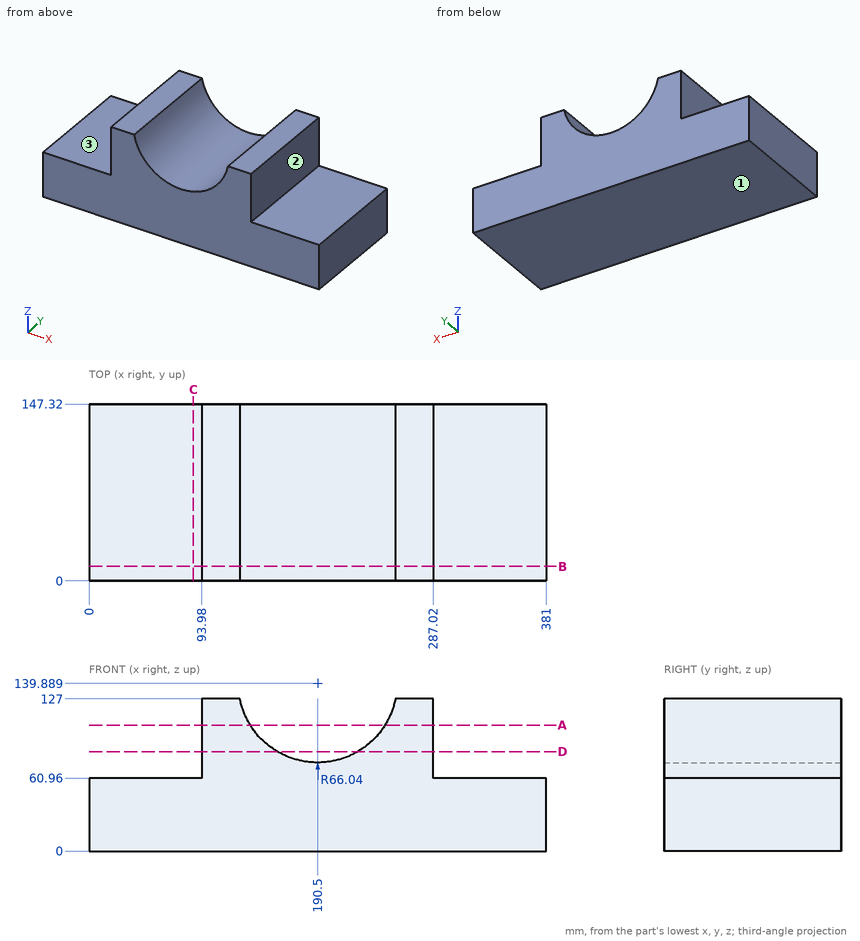
Verification items for this drawing (mm, ordinates from the low corner). A direction names the side the tool comes from. Coordinates: 2 decimals unless noted, no trailing zeros. Order: outer loops, then holes, each group sorted by start corner. A loop starts at its lowest first (then second) coordinate and runs counter-clockwise, first axis right, second up. Notation, with made-up numbers: (65.25, 25.25) - (76.25, 25.25) arc R23 ccw to (76.25, 57.25) - close; hole circle Ø8 at (74.5, 50.25). An arc over 180 degrees is marked (long way). Answer as a JSON object with one key per item and string values. Group by question number.
Item 1: Sectioned sample at C-C, the plane x = 87. Record the cut outline in (y, z).
Item 2: Sectioned sample at D-D, the plane z = 83. Record the cut outline in (x, y), and give its area (3 significant figures).
Item 3: Sectioned sample at B-B, the plane y = 12. Record the cut outline in (x, z).
Item 4: Sectioned sample at A-A, the plane z = 105. Record the cut outline in (x, y).
Item 5: Tool access check on the marked faces 1, 2 and 3. Record the directions out of +Z, -Z, +X, -X, +Y, -Y that give a thin tool (end or side, any length) a straight path to the whole face; none if there is none.
Item 6: Depth check by flat-ended pin: pin 1 Ø4 at (x, y) = (59, 21.5) entering from +Z; pin 2 Ø6 at (y, z) = (18, 68.5) entering from +X; pin 3 Ø20 at (y, z) = (45.5, 95.5) entering from -X. Enter the tip coordinate at first touch or a pass-through.
Item 7: Scan lines: probe 1 along Z at (x, y) = (291, 45); probe 2 along X at (y, z) = (121.5, 108.5); probe 3 along X at (y, z) = (67, 99). Record each from-to range of solid material in increasing order.
Resolved:
{
 "1": {"outline": "(0, 0) - (147.32, 0) - (147.32, 60.96) - (0, 60.96) - close"},
 "2": {"outline": "(93.98, 0) - (156.96, 0) - (156.96, 147.32) - (93.98, 147.32) - close; (224.04, 0) - (287.02, 0) - (287.02, 147.32) - (224.04, 147.32) - close", "area": "18,600 mm^2"},
 "3": {"outline": "(0, 0) - (381, 0) - (381, 60.96) - (287.02, 60.96) - (287.02, 127) - (255.27, 127) arc R66.04 cw to (125.73, 127) - (93.98, 127) - (93.98, 60.96) - (0, 60.96) - close"},
 "4": {"outline": "(93.98, 0) - (134.43, 0) - (134.43, 147.32) - (93.98, 147.32) - close; (246.57, 0) - (287.02, 0) - (287.02, 147.32) - (246.57, 147.32) - close"},
 "5": {"face 1": "-Z, +X, -X, +Y, -Y", "face 2": "+Z, +X, +Y, -Y", "face 3": "+Z, -X, +Y, -Y"},
 "6": {"pin 1": "z = 60.96", "pin 2": "x = 287.02", "pin 3": "x = 93.98"},
 "7": {"probe 1": "0 to 60.96", "probe 2": "93.98 to 132.4, 248.6 to 287.02", "probe 3": "93.98 to 138.64, 242.36 to 287.02"}
}
